For this review, use the dimensioned drawing (mm, ordinates from the lowest corner) and the shaded views. Round coordinates to 2 decimals unless told otherwise and drop trailing zeros. Order: outer loops, then holes, each group sorted by start corner. A loop starts at its lowest first (then second) coordinate and runs counter-clockwise, first axis right, second up. Notation, with made-up numbers: (58.25, 88) - (109.25, 88) arc R34 ccw to (109.25, 127) - close; hole circle Ø4 at (39.25, 77). An arc over 180 degrees is marked (long way). Write item = value, one per line.
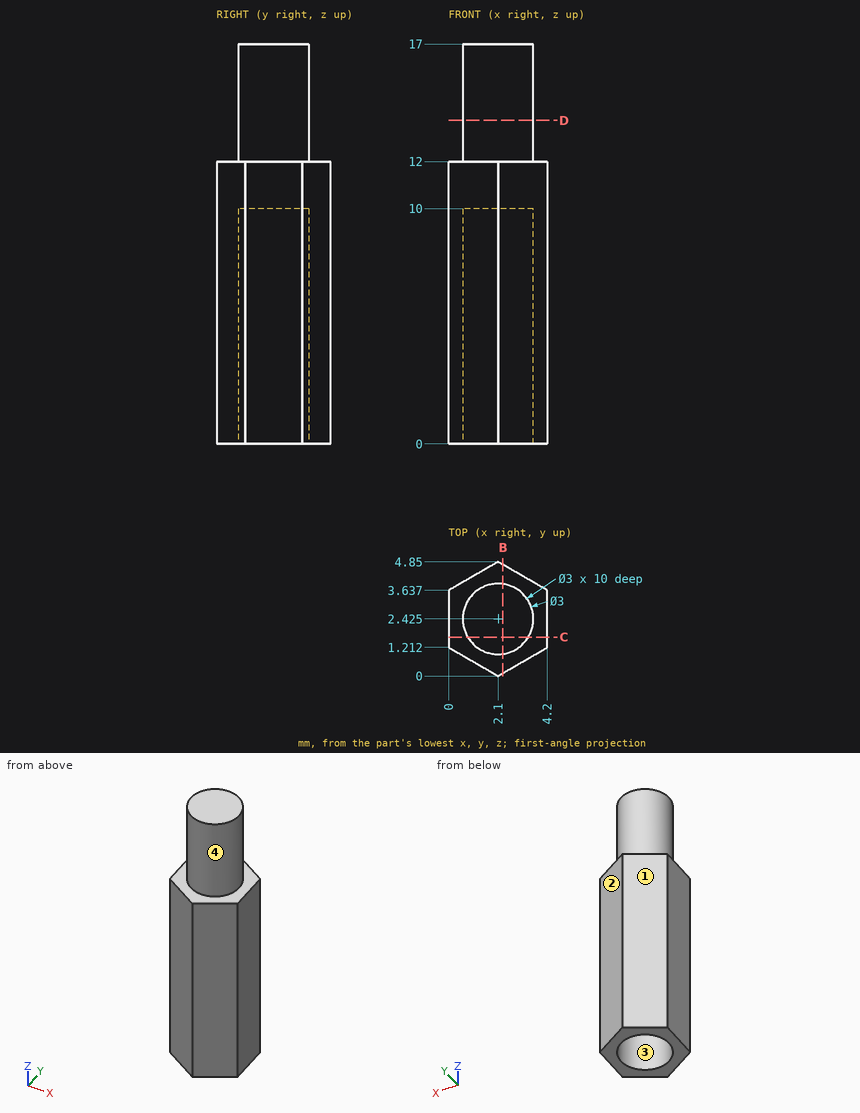
1) We need section B-B on x = 2.3. Write out the cut boundary in (y, z) (1 decimal).
Findings:
outline = (0.1, 0) - (0.9, 0) - (0.9, 10) - (3.9, 10) - (3.9, 0) - (4.7, 0) - (4.7, 12) - (3.9, 12) - (3.9, 17) - (0.9, 17) - (0.9, 12) - (0.1, 12) - close
2) We need section D-D on z = 13.75. Write out the cut boundary in (x, y) (1 decimal).
Findings:
outline = circle Ø3 at (2.1, 2.4)
3) Clearance check with flat-ended pins moving along their axes: pin 1 Ø2.5 at (x, y) = (2.5, 2.5) entering from -Z; pin 2 Ø2 at (y, z) = (1.5, 13.5) entering from -X. State where each tip first meets the part, or that it passes through.
Findings:
pin_1 = 0
pin_2 = 0.6
4) To check wall thickness, follow L1, parallel to X at y = 2.4, z = 2.75; L2, parallel to Z at x = 1.5, y = 0.9; L3, parallel to X at y = 3.8, z = 8.5 (1 decimal). State the ranges of each line that lie inside material, in increasing order. Write a range as from..to.
Findings:
L1 = 0..0.6, 3.6..4.2
L2 = 0..12
L3 = 0.3..1.5, 2.7..3.9
5) The part is to be moulded in two halves that separate along X. For the marked faces 1, 2, 3 and 4, say which applies: released by +X, released by -X, zero draft, split by the parting line, or undercut.
Findings:
face_1 = released by -X
face_2 = released by +X
face_3 = undercut
face_4 = split by the parting line
6) We need section C-C on y = 1.65. Write out the cut boundary in (x, z) (1 decimal).
Findings:
outline = (0, 0) - (0.8, 0) - (0.8, 10) - (3.4, 10) - (3.4, 0) - (4.2, 0) - (4.2, 12) - (3.4, 12) - (3.4, 17) - (0.8, 17) - (0.8, 12) - (0, 12) - close
